Autodesk Inventor part; units mm, degrees
ref_plane "Начальная плоскость" through (0, 0, 46) normal (0, 0, 1) x (1, 0, 0)
ref_plane "Конечная плоскость" through (0, 0, 161.172) normal (0, 0, 1) x (1, 0, 0)
ref_plane "РабПлоскость8" through (-1308.544, -50, 46) normal (0, 0, -1) x (-1, 0, 0)
ref_plane "Начальная плоскость" through (0, 0, 46) normal (0, 0, 1) x (1, 0, 0)
ref_plane "Конечная плоскость" through (0, 0, 161.172) normal (0, 0, 1) x (1, 0, 0)
sketch "Эскиз" plane through (0, 0, 0) normal (0, 0, 1) x (1, 0, 0)
  line L0 (46, -50) -> (0, -50)
  line L1 (46, -50) -> (46, -46.6496)
  line L2 (43.2392, -43.6591) -> (10.9418, -41.0753)
  line L3 (4.5, -34.0976) -> (4.5, 34.0976)
  line L4 (43.2392, 43.6591) -> (10.9418, 41.0753)
  line L5 (46, 46.6496) -> (46, 50)
  line L6 (0, 50) -> (46, 50)
  line L7 (0, -50) -> (0, 50)
  arc A0 (4.5, -34.0976) -> (10.9418, -41.0753) centre (11.5, -34.0976) ccw
  arc A1 (10.9418, 41.0753) -> (4.5, 34.0976) centre (11.5, 34.0976) ccw
  arc A2 (46, -46.6496) -> (43.2392, -43.6591) centre (43, -46.6496) ccw
  arc A3 (43.2392, 43.6591) -> (46, 46.6496) centre (43, 46.6496) ccw
  line L8 (0, 70) -> (0, -70) construction
  line L9 (-9.3169, 0) -> (55.9016, 0) construction
  point P0 (46, -43.88)
  point P1 (4.5, -40.56)
  point P2 (4.5, 40.56)
  point P3 (46, 43.88)
  dimension "d3" = 46
  dimension "d5" = 4.5
  dimension "d7" = 100
  dimension "d9" = 9.44
  dimension "d11" = 9.44
  dimension "d13" = 6.12
  dimension "d15" = 6.12
  dimension "d22" = 7
  dimension "d23" = 3
  dimension "d24" = 50
  dimension "d25" = 0
extrude "Тело" add sketch "Эскиз" along normal up to surface (115.172 mm away) from surface at 46
sketch "Sketch3" plane through (0, 0, 0) normal (0, 0, 1) x (1, 0, 0)
  line L0 (0, 0) -> (10, 0)
ref_plane "Work Plane7" through (0, 0, 0) normal (0, -1, 0) x (1, 0, 0)
sketch "Sketch4" plane through (0, 0, 0) normal (0, -1, 0) x (1, 0, 0)
  line L0 (-2, 46) -> (12, 46)
  line L1 (-2, 161.172) -> (12, 161.172)
  dimension "d29" = 115.172
ref_plane "РабПлоскость8" through (-1308.544, -50, 46) normal (0, 0, -1) x (-1, 0, 0)
split "Разделение1" plane through (-1308.544, -50, 46) removes the side toward (0, 0, -1)
ref_plane "РабПлоскость9" through (46, -50, 161.172) normal (0, 0, 1) x (1, 0, 0)
split "Разделение2" plane through (46, -50, 161.172) removes the side toward (0, 0, 1)
equation "\"d3\" = b"
equation "\"d7\" = ParH"
equation "\"d22\" = R"
equation "\"d23\" = R1"
equation "\"d24\" = 0.5 * d7"
equation "\"d16\" = G_L"
equation "\"R1\" = 3"
equation "\"R\" = 7"
equation "\"t1\" = 4.5"
equation "\"t2\" = 7.6"
equation "\"ParH\" = 100"
equation "\"b\" = 46"
equation "\"msp_x1\" = 0.04 * b"
equation "\"msp_x2\" = -0.08 * t1 + 0.04 * b"
equation "\"G_L\" = d29"
equation "\"ex\" = 0"
equation "\"G_OFFSET_START\" = -46"
equation "\"G_OFFSET_END\" = -46"
equation "\"d26\" = -G_OFFSET_START"
equation "\"d27\" = G_OFFSET_END + B_L"
equation "\"B_L\" = 207.172"
properties part number "Швеллер 10U-115,17 ГОСТ 8240-97" material "Сталь, мягкая"
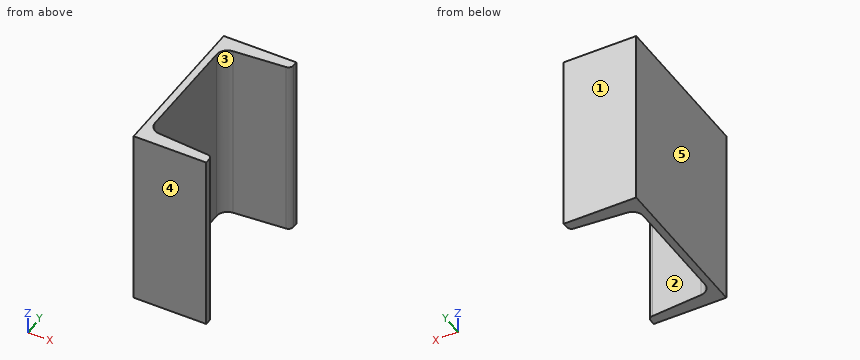
Can you work these out from the model? Positions are in its coordinate system, mm. Face numbers are marked on the shaded views. A direction names the side the tool comes from. Coordinates: 2 decimals unless noted, no trailing zeros. Loops run counter-clockwise (first coordinate to the right, second up) from the corner with the lowest first, then second, coordinate; pieces in that order, holes last. Notation, with made-up numbers: (41.25, 45.25) - (47.25, 45.25) arc R21 cw to (47.25, 72.25) - close; hole circle Ø1 at (31, 27.25). An arc over 180 degrees is marked (long way). Use a Markdown table: item, result.
Item 1: I want a section at B-B on z = 134. Please give me the cut outline in (x, y), and give its area (3 significant figures).
Numbers:
| item | result |
|---|---|
| outline | (0, -50) - (46, -50) - (46, -46.65) arc R3 ccw to (43.24, -43.66) - (10.94, -41.08) arc R7 cw to (4.5, -34.1) - (4.5, 34.1) arc R7 cw to (10.94, 41.08) - (43.24, 43.66) arc R3 ccw to (46, 46.65) - (46, 50) - (0, 50) - close |
| area | 1,110 mm2 |
Item 2: I want a section at C-C on y = 3. Please give me the cut outline in (x, z), and give its area (3 significant figures).
Numbers:
| item | result |
|---|---|
| outline | (0, 46) - (4.5, 46) - (4.5, 161.17) - (0, 161.17) - close |
| area | 518 mm2 |
Item 3: I want a section at A-A on x = 24.5. Please give me the cut outline in (y, z), and give its area (3 significant figures).
Numbers:
| item | result |
|---|---|
| outline | (-50, 46) - (-42.16, 46) - (-42.16, 161.17) - (-50, 161.17) - close; (42.16, 46) - (50, 46) - (50, 161.17) - (42.16, 161.17) - close |
| area | 1,810 mm2 |
Item 4: We'd pull the mould along Y, two halves only. Please class the marked faces 3, 4 and 5: released by +Y, released by -Y, zero draft, split by the parting line, or undercut.
Numbers:
| item | result |
|---|---|
| face 3 | undercut |
| face 4 | released by -Y |
| face 5 | zero draft |
Item 5: I want a section at D-D on x = 9. Please give me the cut outline in (y, z), and give its area (3 significant figures).
Numbers:
| item | result |
|---|---|
| outline | (-50, 46) - (-40.64, 46) - (-40.64, 161.17) - (-50, 161.17) - close; (40.64, 46) - (50, 46) - (50, 161.17) - (40.64, 161.17) - close |
| area | 2,160 mm2 |
Item 6: If I drill on probe 1 along X at (y, z) = (-28.5, 93.5); probe 2 along Y at (x, z) = (37.5, 92); probe 3 along Y at (x, z) = (16.5, 91.5), over which ranges is the centre line in solid material (lowest first)? Write a range as from..to.
Numbers:
| item | result |
|---|---|
| probe 1 | x = 0..4.5 |
| probe 2 | y = -50..-43.2, 43.2..50 |
| probe 3 | y = -50..-41.52, 41.52..50 |
Item 7: For the marked faces 1 and 2, which set-ups out of +Z, -Z, +X, -X, +Y, -Y let a thin tool reach every point of the face, with its end or its side?
Numbers:
| item | result |
|---|---|
| face 1 | +Z, -Z, +X, -X, +Y |
| face 2 | +Z, -Z, +X |
Item 8: Will these pins go through, and if not, where does the flat tip stop? pin 1 (2 mm diameter, centred on y = -34, z = 96, fed in from +X); pin 2 (4 mm diameter, centred on y = 37, z = 119, fed in from +X).
Numbers:
| item | result |
|---|---|
| pin 1 | stops at x = 4.56 |
| pin 2 | stops at x = 6.5 |
